Geometry check sheet. Reference: the model listing, model coordinates, mm. Face numbers are marked on the shaded views. A direction names the side the tool comes from. Coordinates: 2 decimals unless noted, no trailing zeros. Write each loop counter-clockwise with the first axis right and the second up, starting at its lowest first coordinate (ties: lowest second). Pieces come first, ordered by that corner, then holes.
from build123d import *

# Parameters (mm, degrees)
SKETCH1_R                  = 32.004
BOSS_EXTRUDE1_DEPTH        = 68.7568
SKETCH2_R                  = 31.877
BOSS_EXTRUDE2_DEPTH        = 8.2296
SKETCH3_R                  = 15.0368
BOSS_EXTRUDE3_DEPTH        = 5
BOSS_EXTRUDE4_START        = 8.2296
SKETCH4_R                  = 31.877
BOSS_EXTRUDE4_DEPTH        = 8.2296
SKETCH5_R                  = 9.525
BOSS_EXTRUDE5_DEPTH        = 4
SKETCH6_R                  = 4
BOSS_EXTRUDE6_DEPTH        = 31.6
CUT_EXTRUDE1_REACH         = 103.855
CUT_EXTRUDE1_END_RADIUS    = 4
F_10_32_TAPPED_HOLE1_D     = 4.0386
F_10_32_TAPPED_HOLE1_DEPTH = 12.03
F_10_32_TAPPED_HOLE1_TIP   = 1.213317848
CHAMFER1_SIZE              = 1.016
CHAMFER2_SIZE              = 0.5
FILLET1_R                  = 1


with BuildPart() as part:
    # Sketch1 → Boss-Extrude1 (new body)
    with BuildSketch(Plane(origin=(8.2296, 0, 0), x_dir=(0, -1, 0), z_dir=(-1, 0, 0))):
        with Locations(Location((0, 0, 0), (0, 0, 270))):
            Circle(SKETCH1_R)
    extrude(amount=-BOSS_EXTRUDE1_DEPTH)

    # Sketch2 → Boss-Extrude2 (add)
    with BuildSketch(Plane(origin=(76.9864, 0, 0), x_dir=(0, 0, -1), z_dir=(1, 0, 0))):
        Circle(SKETCH2_R)
    extrude(amount=BOSS_EXTRUDE2_DEPTH)

    # Sketch3 → Boss-Extrude3 (add)
    with BuildSketch(Plane(origin=(85.216, 0, 0), x_dir=(0, 0, -1), z_dir=(1, 0, 0))):
        Circle(SKETCH3_R)
    extrude(amount=BOSS_EXTRUDE3_DEPTH)

    # Sketch4 → Boss-Extrude4 (add)
    with BuildSketch(Plane.ZY.offset(-8.2296).offset(BOSS_EXTRUDE4_START)):
        with Locations(Location((0, 0, 0), (0, 0, 180))):
            Circle(SKETCH4_R)
    extrude(amount=-BOSS_EXTRUDE4_DEPTH)

    # Sketch5 → Boss-Extrude5 (add)
    with BuildSketch(Plane.ZY):
        Circle(SKETCH5_R)
    extrude(amount=BOSS_EXTRUDE5_DEPTH)

    # Sketch6 → Boss-Extrude6 (add)
    with BuildSketch(Plane.ZY.offset(4)):
        Circle(SKETCH6_R)
    extrude(amount=BOSS_EXTRUDE6_DEPTH)

    # Cut-Extrude1: up to this cylinder (the profile starts inside it)
    cut_extrude1_end = Plane(origin=(-16.85, 0, 0), z_dir=(1, 0, 0)) * Cylinder(CUT_EXTRUDE1_END_RADIUS, 216.71, mode=Mode.PRIVATE)
    # Sketch7 → Cut-Extrude1 (cut, up to the surface)
    with BuildSketch(Plane.XZ.offset(-2.8), mode=Mode.PRIVATE) as cut_extrude1_sk1:
        with BuildLine():
            Line((-7.1, 1), (-26.6, 1))
            ThreePointArc((-26.6, 1), (-27.6, 0), (-26.6, -1))
            Line((-26.6, -1), (-7.1, -1))
            ThreePointArc((-7.1, -1), (-6.1, 0), (-7.1, 1))
        make_face()
    cut_extrude1_tool1 = extrude(cut_extrude1_sk1.sketch, amount=-CUT_EXTRUDE1_REACH, mode=Mode.PRIVATE) & cut_extrude1_end
    add(cut_extrude1_tool1.solids().sort_by_distance((-16.85, 2.8, 0))[0], mode=Mode.SUBTRACT)

    # Sketch8 → Revolve1 (revolve)
    with BuildSketch(Plane.XY.offset(-18.607090683), mode=Mode.PRIVATE) as revolve1_sk:
        Polygon((85.216, 15.525359639), (85.216, 11.207359639), (87.4639, 11.207359639), (87.4639, 13.325359639), (85.2639, 15.525359639), align=None)
    revolve(revolve1_sk.sketch.rotate(Axis((85.216, 11.207359639, -18.607090683), (1, 0, 0)), 270), axis=Axis((85.216, 11.207359639, -18.607090683), (1, 0, 0)))

    # Sketch9 → Revolve2 (revolve)
    with BuildSketch(Plane.XY.offset(-11.207359639), mode=Mode.PRIVATE) as revolve2_sk:
        Polygon((85.216, 22.925090683), (85.216, 18.607090683), (87.4639, 18.607090683), (87.4639, 20.725090683), (85.2639, 22.925090683), align=None)
    revolve(revolve2_sk.sketch.rotate(Axis((85.216, 18.607090683, -11.207359639), (1, 0, 0)), 270), axis=Axis((85.216, 18.607090683, -11.207359639), (1, 0, 0)))

    # #10-32 Tapped Hole1
    with Locations(Plane.ZY):
        with Locations((0, 25.4), (0, -25.4)):
            Hole(F_10_32_TAPPED_HOLE1_D / 2, depth=F_10_32_TAPPED_HOLE1_DEPTH)
            with Locations((0, 0, -(F_10_32_TAPPED_HOLE1_DEPTH + F_10_32_TAPPED_HOLE1_TIP / 2))):  # 118° drill point
                Cone(0, F_10_32_TAPPED_HOLE1_D / 2, F_10_32_TAPPED_HOLE1_TIP, mode=Mode.SUBTRACT)

    # Chamfer1
    chamfer1_edges = [part.edges().sort_by_distance(p)[0] for p in [
        (90.216, 0, 15.0368),
        (-4, 0, -9.525),
    ]]
    chamfer(chamfer1_edges, length=CHAMFER1_SIZE)

    # Chamfer2
    chamfer2_edges = [part.edges().sort_by_distance(p)[0] for p in [
        (-35.6, 0, -4),
    ]]
    chamfer(chamfer2_edges, length=CHAMFER2_SIZE)

    # Fillet1
    fillet1_edges = [part.edges().sort_by_distance(p)[0] for p in [
        (0, 0, 31.877),
        (85.216, 0, 31.877),
    ]]
    fillet(fillet1_edges, radius=FILLET1_R)


solid = part.part
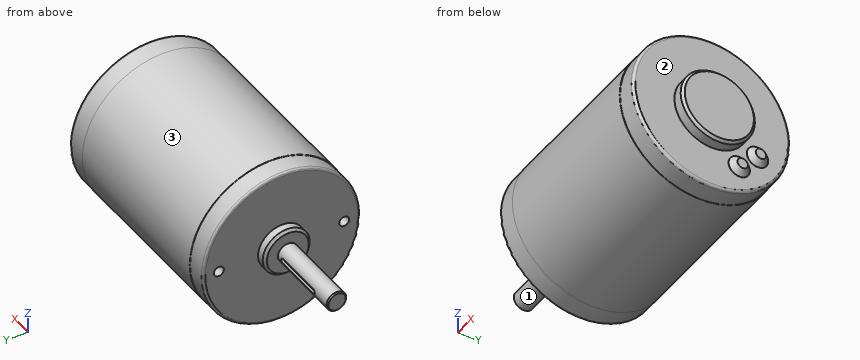
1. Access from +Z, -Z, +X, -X, +Y, -Y to the whole of each face (thin tool, end or side, straight path). Record for the marked faces 1, 2 and 3.
Computed values:
face 1: -X
face 2: +X
face 3: +X, -X
2. Thickness scan on line 1 along Y through (x, z) = (4.5, 0); line 2 along X through (y, z) = (-5, -0.5); line 3 along Z through (x, y) = (6.5, -25.4). Record the ranges inside material, lowest first.
Computed values:
line 1: y = -31.88 to -27.42, -23.38 to 23.38, 27.42 to 31.88
line 2: x = -4 to 90.22
line 3: z = -19.26 to -2.02, 2.02 to 19.26
3. Sectioned sample at C-C, the plane x = -10. Record the boundary of the cut face in (y, z), and give its area (3 significant figures).
Computed values:
outline: (2.8, -1) - (2.8, 1) - (3.87, 1) arc R4 ccw (long way) to (3.87, -1) - close
area: 47.9 mm2
4. Gauge pin test, flat ends, axial feed: pin 1 Ø1.2 at (x, y) = (-18, 3.5) entering from +Z (3 decimals); pin 2 Ø13.5 at (y, z) = (3.5, 2) entering from -X; pin 3 Ø10 at (x, z) = (70.5, -4) entering from -Y; pin 4 Ø19 at (y, z) = (6.5, 14.5) entering from -X. Record the tip position at first contact, or that the pin passes through.
Computed values:
pin 1: stops at z = 2.755
pin 2: stops at x = -35.6
pin 3: stops at y = -32
pin 4: stops at x = -4
5. Sectioned sample at B-B, the plane x = 37.5. Record the boundary of the cut face in (y, z), and give its area (3 significant figures).
Computed values:
outline: circle Ø64.01 at (0, 0)
area: 3,220 mm2
